```python
from build123d import *

# Parameters (mm, degrees)
BOSS_EXTRUDE1_DEPTH = 1.5
FILLET1_R           = 0.5
BOSS_EXTRUDE2_START = 5
SKETCH2_R           = 9
SKETCH2_R_2         = 7.5
BOSS_EXTRUDE2_DEPTH = 5


with BuildPart() as part:
    # Sketch1 → Boss-Extrude1 (new body)
    with BuildSketch(Plane(origin=(0, 0, 0), x_dir=(1, 0, 0), z_dir=(0, 1, 0))):
        with BuildLine():
            ThreePointArc((0.899416611, 12.4676), (1.956802124, 12.345886985), (3, 12.1346611))
            Line((3, 12.1346611), (3, 12.5))
            ThreePointArc((3, 12.5), (0, 15.5), (-3, 12.5))
            Line((-3, 12.5), (-3, 12.1346611))
            ThreePointArc((-3, 12.1346611), (-1.956802124, 12.345886985), (-0.899416611, 12.4676))
            ThreePointArc((-0.899416611, 12.4676), (-0.016202626, 13.399854141), (0.9, 12.5))
            ThreePointArc((0.9, 12.5), (0.899854141, 12.483797374), (0.899416611, 12.4676))
        make_face()
        with BuildLine():
            ThreePointArc((-3, 6.873863542), (0, 7.5), (3, 6.873863542))
            Line((3, 6.873863542), (3, 12.1346611))
            ThreePointArc((3, 12.1346611), (1.956802124, 12.345886985), (0.899416611, 12.4676))
            ThreePointArc((0.899416611, 12.4676), (0, 11.6), (-0.899416611, 12.4676))
            ThreePointArc((-0.899416611, 12.4676), (-1.956802124, 12.345886985), (-3, 12.1346611))
            Line((-3, 12.1346611), (-3, 6.873863542))
        make_face()
        with BuildLine():
            Line((3, 12.1346611), (3, 6.873863542))
            ThreePointArc((3, 6.873863542), (4.565710718, 5.950150052), (5.863185187, 4.676864277))
            Line((5.863185187, 4.676864277), (10.944725414, 6.038458877))
            ThreePointArc((10.944725414, 6.038458877), (7.609517863, 9.916916754), (3, 12.1346611))
        make_face()
        with BuildLine():
            ThreePointArc((7.5, 0), (7.48822587, -0.420087268), (7.45294045, -0.83885556))
            Line((7.45294045, -0.83885556), (7.772310826, -1.023244132))
            Line((7.772310826, -1.023244132), (12.497639685, 0.24290392))
            ThreePointArc((12.497639685, 0.24290392), (12.43679381, 1.255451998), (12.294047703, 2.259732526))
            ThreePointArc((12.294047703, 2.259732526), (11.108147002, 2.976419019), (11.776823889, 4.190038078))
            ThreePointArc((11.776823889, 4.190038078), (11.39830538, 5.131143582), (10.944725414, 6.038458877))
            Line((10.944725414, 6.038458877), (5.863185187, 4.676864277))
            ThreePointArc((5.863185187, 4.676864277), (7.078979054, 2.477509949), (7.5, 0))
        make_face()
        with BuildLine():
            ThreePointArc((12.294047703, 2.259732526), (12.43679381, 1.255451998), (12.497639685, 0.24290392))
            Line((12.497639685, 0.24290392), (12.850529964, 0.337460585))
            ThreePointArc((12.850529964, 0.337460585), (14.971850307, 4.011695199), (11.297615693, 6.133015543))
            Line((11.297615693, 6.133015543), (10.944725414, 6.038458877))
            ThreePointArc((10.944725414, 6.038458877), (11.39830538, 5.131143582), (11.776823889, 4.190038078))
            ThreePointArc((11.776823889, 4.190038078), (12.666842202, 4.040610319), (13.074072829, 3.235238064))
            ThreePointArc((13.074072829, 3.235238064), (12.855089754, 2.610728206), (12.294047703, 2.259732526))
        make_face()
        with BuildLine():
            Line((12.497639685, 0.24290392), (7.772310826, -1.023244132))
            Line((7.772310826, -1.023244132), (12.008924778, -3.469254338))
            ThreePointArc((12.008924778, -3.469254338), (12.376622312, -1.751918986), (12.5, 0))
            ThreePointArc((12.5, 0), (12.499409907, 0.121457693), (12.497639685, 0.24290392))
        make_face()
        with BuildLine():
            ThreePointArc((7.45294045, -0.83885556), (7.43583646, -0.978946442), (7.416099457, -1.118690681))
            Line((7.416099457, -1.118690681), (7.772310826, -1.023244132))
            Line((7.772310826, -1.023244132), (7.45294045, -0.83885556))
        make_face()
        with BuildLine():
            Line((7.772310826, -1.023244132), (7.416099457, -1.118690681))
            ThreePointArc((7.416099457, -1.118690681), (6.42347811, -3.871553818), (4.45294045, -6.035007983))
            Line((4.45294045, -6.035007983), (9.008924778, -8.665406761))
            ThreePointArc((9.008924778, -8.665406761), (9.713450699, -7.867583842), (10.347550019, -7.012717634))
            ThreePointArc((10.347550019, -7.012717634), (10.045894684, -5.8), (11.24696663, -5.454882366))
            ThreePointArc((11.24696663, -5.454882366), (11.670252823, -4.478303143), (12.008924778, -3.469254338))
            Line((12.008924778, -3.469254338), (7.772310826, -1.023244132))
        make_face()
        with BuildLine():
            ThreePointArc((10.347550019, -7.012717634), (9.713450699, -7.867583842), (9.008924778, -8.665406761))
            Line((9.008924778, -8.665406761), (9.325317547, -8.848076211))
            ThreePointArc((9.325317547, -8.848076211), (13.423393759, -7.75), (12.325317547, -3.651923789))
            Line((12.325317547, -3.651923789), (12.008924778, -3.469254338))
            ThreePointArc((12.008924778, -3.469254338), (11.670252823, -4.478303143), (11.24696663, -5.454882366))
            ThreePointArc((11.24696663, -5.454882366), (11.59651278, -5.786041044), (11.725317547, -6.25))
            ThreePointArc((11.725317547, -6.25), (11.261212732, -7.037397859), (10.347550019, -7.012717634))
        make_face()
        with BuildLine():
            ThreePointArc((4.45294045, -6.035007983), (3.75, -6.495190528), (3, -6.873863542))
            Line((3, -6.873863542), (3, -12.1346611))
            ThreePointArc((3, -12.1346611), (6.25, -10.825317547), (9.008924778, -8.665406761))
            Line((9.008924778, -8.665406761), (4.45294045, -6.035007983))
        make_face()
        with BuildLine():
            Line((3, -12.1346611), (3, -6.873863542))
            ThreePointArc((3, -6.873863542), (0, -7.5), (-3, -6.873863542))
            Line((-3, -6.873863542), (-3, -12.1346611))
            ThreePointArc((-3, -12.1346611), (-2.00620559, -12.337955225), (-0.99919968, -12.46))
            ThreePointArc((-0.99919968, -12.46), (0, -11.5), (0.99919968, -12.46))
            ThreePointArc((0.99919968, -12.46), (2.00620559, -12.337955225), (3, -12.1346611))
        make_face()
        with BuildLine():
            Line((3, -12.5), (3, -12.1346611))
            ThreePointArc((3, -12.1346611), (2.00620559, -12.337955225), (0.99919968, -12.46))
            ThreePointArc((0.99919968, -12.46), (0.9997999, -12.479995997), (1, -12.5))
            ThreePointArc((1, -12.5), (-0.020004003, -13.4997999), (-0.99919968, -12.46))
            ThreePointArc((-0.99919968, -12.46), (-2.00620559, -12.337955225), (-3, -12.1346611))
            Line((-3, -12.1346611), (-3, -12.5))
            ThreePointArc((-3, -12.5), (0, -15.5), (3, -12.5))
        make_face()
        with BuildLine():
            Line((-3, -12.1346611), (-3, -6.873863542))
            ThreePointArc((-3, -6.873863542), (-3.75, -6.495190528), (-4.45294045, -6.035007983))
            Line((-4.45294045, -6.035007983), (-9.008924778, -8.665406761))
            ThreePointArc((-9.008924778, -8.665406761), (-6.25, -10.825317547), (-3, -12.1346611))
        make_face()
        with BuildLine():
            Line((-9.008924778, -8.665406761), (-4.45294045, -6.035007983))
            ThreePointArc((-4.45294045, -6.035007983), (-6.42347811, -3.871553818), (-7.416099457, -1.118690681))
            Line((-7.416099457, -1.118690681), (-7.772310826, -1.023244132))
            Line((-7.772310826, -1.023244132), (-12.008924778, -3.469254338))
            ThreePointArc((-12.008924778, -3.469254338), (-11.670252823, -4.478303143), (-11.24696663, -5.454882366))
            ThreePointArc((-11.24696663, -5.454882366), (-10.361358591, -5.478804767), (-9.925317547, -6.25))
            ThreePointArc((-9.925317547, -6.25), (-10.037919689, -6.685895185), (-10.347550019, -7.012717634))
            ThreePointArc((-10.347550019, -7.012717634), (-9.713450699, -7.867583842), (-9.008924778, -8.665406761))
        make_face()
        with BuildLine():
            Line((-9.325317547, -8.848076211), (-9.008924778, -8.665406761))
            ThreePointArc((-9.008924778, -8.665406761), (-9.713450699, -7.867583842), (-10.347550019, -7.012717634))
            ThreePointArc((-10.347550019, -7.012717634), (-11.604740411, -6.7), (-11.24696663, -5.454882366))
            ThreePointArc((-11.24696663, -5.454882366), (-11.670252823, -4.478303143), (-12.008924778, -3.469254338))
            Line((-12.008924778, -3.469254338), (-12.325317547, -3.651923789))
            ThreePointArc((-12.325317547, -3.651923789), (-13.423393759, -7.75), (-9.325317547, -8.848076211))
        make_face()
        with BuildLine():
            Line((-7.772310826, -1.023244132), (-7.416099457, -1.118690681))
            ThreePointArc((-7.416099457, -1.118690681), (-7.43583646, -0.978946442), (-7.45294045, -0.83885556))
            Line((-7.45294045, -0.83885556), (-7.772310826, -1.023244132))
        make_face()
        with BuildLine():
            Line((-12.008924778, -3.469254338), (-7.772310826, -1.023244132))
            Line((-7.772310826, -1.023244132), (-12.497639685, 0.24290392))
            ThreePointArc((-12.497639685, 0.24290392), (-12.393060767, -1.631577403), (-12.008924778, -3.469254338))
        make_face()
        with BuildLine():
            ThreePointArc((-7.45294045, -0.83885556), (-7.206635264, 2.07711535), (-5.863185187, 4.676864277))
            Line((-5.863185187, 4.676864277), (-10.944725414, 6.038458877))
            ThreePointArc((-10.944725414, 6.038458877), (-11.39830538, 5.131143582), (-11.776823889, 4.190038078))
            ThreePointArc((-11.776823889, 4.190038078), (-11.268700573, 3.828007437), (-11.074072829, 3.235238064))
            ThreePointArc((-11.074072829, 3.235238064), (-11.44956297, 2.454221139), (-12.294047703, 2.259732526))
            ThreePointArc((-12.294047703, 2.259732526), (-12.43679381, 1.255451998), (-12.497639685, 0.24290392))
            Line((-12.497639685, 0.24290392), (-7.772310826, -1.023244132))
            Line((-7.772310826, -1.023244132), (-7.45294045, -0.83885556))
        make_face()
        with BuildLine():
            ThreePointArc((-11.776823889, 4.190038078), (-11.39830538, 5.131143582), (-10.944725414, 6.038458877))
            Line((-10.944725414, 6.038458877), (-11.297615693, 6.133015543))
            ThreePointArc((-11.297615693, 6.133015543), (-14.971850307, 4.011695199), (-12.850529964, 0.337460585))
            Line((-12.850529964, 0.337460585), (-12.497639685, 0.24290392))
            ThreePointArc((-12.497639685, 0.24290392), (-12.43679381, 1.255451998), (-12.294047703, 2.259732526))
            ThreePointArc((-12.294047703, 2.259732526), (-13.039998655, 3.494057109), (-11.776823889, 4.190038078))
        make_face()
        with BuildLine():
            ThreePointArc((-5.863185187, 4.676864277), (-4.565710718, 5.950150052), (-3, 6.873863542))
            Line((-3, 6.873863542), (-3, 12.1346611))
            ThreePointArc((-3, 12.1346611), (-7.609517863, 9.916916754), (-10.944725414, 6.038458877))
            Line((-10.944725414, 6.038458877), (-5.863185187, 4.676864277))
        make_face()
    extrude(amount=BOSS_EXTRUDE1_DEPTH)

    # Fillet1
    fillet1_edges = [part.edges().sort_by_distance(p)[0] for p in [
        (-3, 0.75, 12.1346611),
        (3, 0.75, 12.1346611),
        (9.008924778, 0.75, 8.665406761),
        (12.008924778, 0.75, 3.469254338),
        (12.497639685, 0.75, -0.24290392),
        (10.944725414, 0.75, -6.038458877),
        (3, 0.75, -12.1346611),
        (-3, 0.75, -12.1346611),
        (-10.944725414, 0.75, -6.038458877),
        (-12.497639685, 0.75, -0.24290392),
        (-12.008924778, 0.75, 3.469254338),
        (-9.008924778, 0.75, 8.665406761),
    ]]
    fillet(fillet1_edges, radius=FILLET1_R)

    # Sketch2 → Boss-Extrude2 (add)
    with BuildSketch(Plane.XZ.offset(BOSS_EXTRUDE2_START)):
        with Locations(Location((0, 0, 0), (0, 0, 90))):
            Circle(SKETCH2_R)
        with Locations(Location((0, 0, 0), (0, 0, 270))):
            Circle(SKETCH2_R_2, mode=Mode.SUBTRACT)
    extrude(amount=-BOSS_EXTRUDE2_DEPTH)


solid = part.part
```
Check sheet for the modelled part. Datum: model origin and axes. Units: mm. A direction names the side the tool comes from. Coordinates: 2 decimals unless noted, no trailing zeros. Loops run counter-clockwise (first coordinate to the right, second up) from the corner with the lowest first, then second, coordinate; pieces in that order, holes last. Notation, with made-up numbers: M 15.5,43 L 35.5,43 A30 cw 35.5,75 Z; hole C 23.25,60 d6. An arc over 180 degrees is marked long. Answer as a JSON object with one key per item and string values.
1. Sectioned sample at A-A on x = 1.5. Record the cut outline in (y, z).
Outcome:
{"outline": "M -5,-8.87 L 0,-8.87 L 0,-15.1 L 1.5,-15.1 L 1.5,-7.35 L -5,-7.35 Z; M -5,7.35 L 1.5,7.35 L 1.5,15.1 L 0,15.1 L 0,8.87 L -5,8.87 Z"}
2. Access from +Z, -Z, +X, -X, +Y, -Y to the whole of each face (thin tool, end or side, straight path). Record for faces 1 (the cylindrical face through (-0.1, 0.7, 15.5)), 2 (the flat face through (-1.2, 0, 9.1)), 3 (the cylindrical face through (-12.396, 0.74, 1.611)).
Outcome:
{"face 1": "+Z, +Y, -Y", "face 2": "-Y", "face 3": "-X, +Y, -Y"}
3. Sectioned sample at D-D on y = -2.75. Record the cut outline in (x, z), and give its area (3 significant figures).
Outcome:
{"outline": "C 0,0 d18; hole C 0,0 d15", "area": "77.8 mm²"}
4. Sectioned sample at B-B on z = -8. Record the cut outline in (x, y), and give its area (3 significant figures).
Outcome:
{"outline": "M -9.6,0 L -4.12,0 L -4.12,-5 L 4.12,-5 L 4.12,0 L 9.6,0 L 9.6,1.5 L -9.6,1.5 Z", "area": "70.0 mm²"}
5. Scan lines: L1, parallel to X at y = -1.25, z = 0; L2, parallel to Z at x = -11.5, y = 1.25; L3, parallel to Y at x = 1, z = -12. Record each from-to range of solid material in increasing order. Write a range as from..to.
Outcome:
{"L1": "-9..-7.5, 7.5..9", "L2": "-6.18..-4.05, -2.42..5.65, 6.85..9.17", "L3": "0..1.5"}
6. Release check for a two-part mould opening along Z. For faces 4 (the cylindrical face through (12.39, 0.74, 1.65)), 5 (the cylindrical face through (6.21, 0.74, 10.85)), 6 (the cylindrical face through (7.66, 0.74, -9.88)) record: pulls with the +Z half, pulls with the -Z half, needs draft (parallel to the pull), parting line crosses it, or undercut.
Outcome:
{"face 4": "undercut", "face 5": "pulls with the +Z half", "face 6": "pulls with the -Z half"}
7. Depth check by flat-ended pin: P1, Ø3, axis at y = -2.5, z = -8.5, coming from the +X side; P2, Ø1, axis at y = -4, z = -6.5, coming from the -X side; P3, Ø8, axis at x = 12, z = -10, coming from the -Y side; P4, Ø1, axis at y = -3, z = -11, coming from the -X side. Enter the tip coordinate at first touch or a pass-through.
Outcome:
{"P1": "x = 5.66", "P2": "x = -6.71", "P3": "y = 0", "P4": "through"}
8. Sectioned sample at C-C on x = 8. Record the cut outline in (y, z), and give its area (3 significant figures).
Outcome:
{"outline": "M -5,-4.12 L 0,-4.12 L 0,-9.6 L 1.5,-9.6 L 1.5,9.6 L 0,9.6 L 0,4.12 L -5,4.12 Z", "area": "70.0 mm²"}
